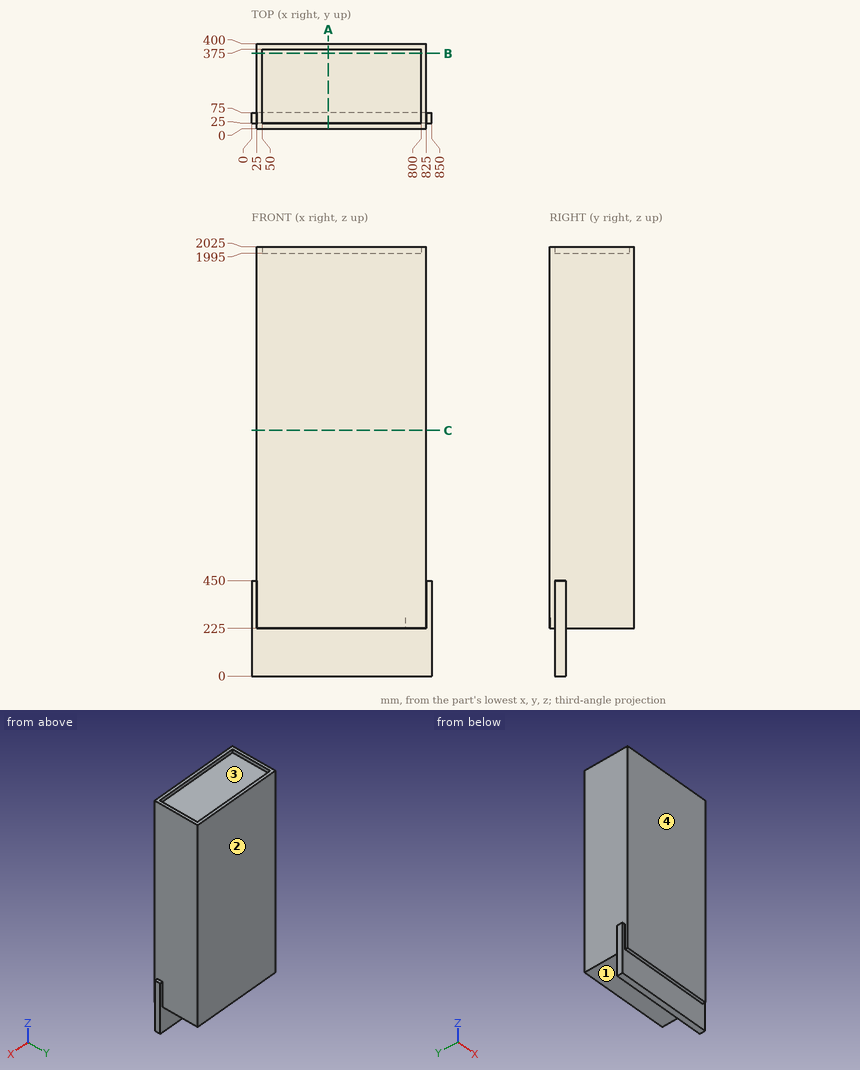
Drawing for the job (mm, zero at the part's lowest x, y, z). A direction names the side the tool comes from. Round coordinates to 2 decimals unless told otherwise and drop trailing zeros. Order: outer loops, then holes, each group sorted by start corner. A loop starts at its lowest first (then second) coordinate and runs counter-clockwise, first axis right, second up. Notation, with made-up numbers: (-13, -21) -> (29, -21) arc R9 cw to (29, -11) -> close; hole circle Ø5 at (1, 68). An arc over 180 degrees is marked (long way). Write item = value, one per line. Start each with the question number.
(1) Cut at C-C, the plane z = 1158.5. List the corners of the cut face in (x, y), then the cut area to 3 significant figures.
(2) Cut at A-A, the plane x = 363. List the corners of the cut face in (y, z).
(3) Pin check, flat tips, straight feed: P1, Ø9, axis at y = 160, z = 2009, coming from the -X side; P2, Ø20, axis at x = 407.5, y = 12.5, coming from the -Z side; P3, Ø4, axis at y = 197, z = 750, coming from the +X side. Stop position of each tip, or through.
(4) Cut at B-B, the plane y = 355.5. List the corners of the cut face in (x, z), then the cut area to 3 significant figures.
(5) Pull direction X, two halves, no side cores. Call the marked faces 3 and 4: released by +X, released by -X, zero draft, split by the parting line, or undercut.
(6) Which spindle directions (+Z, -Z, +X, -X, +Y, -Y) get a long thin tool onto all of the face, cutting with end or side? Do the marked faces 1 and 2. Say none if no direction does.
(7) Probe line 1 (Z direction, x = 435, y = 204); line 2 (X direction, y = 152, z = 1134); line 3 (Z direction, x = 239.5, y = 57). List the from-to ranges inside material, lowest first. Write a range as [from, to].
Model answer:
q1.outline = (25, 0) -> (825, 0) -> (825, 400) -> (25, 400) -> close
q1.area = 320,000 mm2
q2.outline = (0, 225) -> (25, 225) -> (25, 0) -> (75, 0) -> (75, 225) -> (400, 225) -> (400, 2025) -> (375, 2025) -> (375, 1995) -> (25, 1995) -> (25, 2025) -> (0, 2025) -> close
q3.P1 = 25
q3.P2 = 225
q3.P3 = 825
q4.outline = (25, 225) -> (825, 225) -> (825, 2025) -> (800, 2025) -> (800, 1995) -> (50, 1995) -> (50, 2025) -> (25, 2025) -> close
q4.area = 1,420,000 mm2
q5.face_3 = undercut
q5.face_4 = zero draft
q6.face_1 = -Z, +X, -X, +Y
q6.face_2 = +Z, -Z, +X, -X, +Y
q7.line_1 = [225, 1995]
q7.line_2 = [25, 825]
q7.line_3 = [0, 1995]
